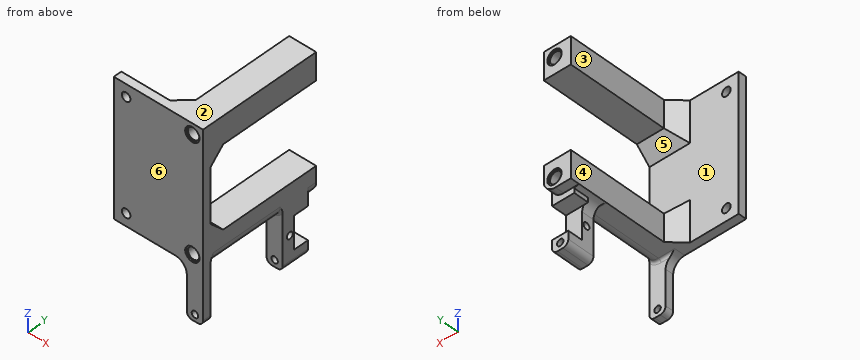
```python
from build123d import *

# Parameters (mm, degrees)
SKETCH1_R           = 1.5999999999999974
SKETCH1_R_2         = 1.6
BOSS_EXTRUDE1_DEPTH = 3
SKETCH2_W           = 10.000000000000004
SKETCH2_H           = 10.000000000000004
BOSS_EXTRUDE2_DEPTH = 42
CHAMFER1_SIZE       = 5
SKETCH3_R           = 2.1
SKETCH3_R_2         = 2.1000000000000005
CUT_EXTRUDE1_DEPTH  = 52.00000000000001
SKETCH4_R           = 2.65
SKETCH4_R_2         = 2.6500000000000004
CUT_EXTRUDE2_DEPTH  = 0.5
BOSS_EXTRUDE3_DEPTH = 14.15
SKETCH6_R           = 1.2000000000000004
CUT_EXTRUDE3_DEPTH  = 6
SKETCH7_W           = 6
SKETCH7_H           = 10.018921584932333
BOSS_EXTRUDE4_DEPTH = 5
BOSS_EXTRUDE5_DEPTH = 2.15
SKETCH9_W           = 6
SKETCH9_H           = 3
BOSS_EXTRUDE6_DEPTH = 19.15
SKETCH10_R          = 1.2000000000000004
CUT_EXTRUDE4_DEPTH  = 64.7666045986287
FILLET3_R           = 2
FILLET4_R           = 4.25
FILLET5_R           = 4.25
FILLET6_R           = 4.25
FILLET7_R           = 4.25
FILLET8_R           = 1
FILLET9_R           = 1


with BuildPart() as part:
    # Sketch1 → Boss-Extrude1 (new body)
    with BuildSketch(Plane(origin=(0, 0, 0), x_dir=(1, 0, 0), z_dir=(0, 1, 0))):
        Polygon((-6.5123966942148765, 9.68595041322314), (1.487603305785124, 9.68595041322314), (26.48760330578513, 9.68595041322314), (26.487603305785132, -40.31404958677687), (1.4876033057851312, -40.31404958677687), (-6.512396694214871, -40.31404958677687), align=None)
        with Locations(Location((-1.962396694214872, -35.76404958677687, 0), (0, 0, 270))):
            Circle(SKETCH1_R, mode=Mode.SUBTRACT)
        with Locations(Location((-1.9623966942148756, 5.135950413223139, 0), (0, 0, 270))):
            Circle(SKETCH1_R_2, mode=Mode.SUBTRACT)
    extrude(amount=BOSS_EXTRUDE1_DEPTH)

    # Sketch2 → Boss-Extrude2 (add)
    with BuildSketch(Plane(origin=(0, 3, 0), x_dir=(1, 0, 0), z_dir=(0, 1, 0))):
        with Locations((21.48760330578513, -35.31404958677687)):
            Rectangle(SKETCH2_W, SKETCH2_H)
        Polygon((26.48760330578513, 9.68595041322314), (16.48760330578513, 9.685950413223138), (16.487603305785125, -0.314049586776863), (26.48760330578513, -0.31404958677686173), align=None)
    extrude(amount=BOSS_EXTRUDE2_DEPTH)

    # Chamfer1
    chamfer1_edges = [part.edges().sort_by_distance(p)[0] for p in [
        (21.48760330578513, 3, 30.314049586776864),
        (16.48760330578513, 3, 35.31404958677687),
        (16.48760330578513, 3, -4.6859504132231375),
        (21.48760330578513, 3, 0.31404958677686234),
    ]]
    chamfer(chamfer1_edges, length=CHAMFER1_SIZE)

    # Sketch3 → Cut-Extrude1 (cut)
    with BuildSketch(Plane(origin=(0, 45.00000000000001, 0), x_dir=(1, 0, 0), z_dir=(0, 1, 0))):
        with Locations(Location((22.53760330578513, -36.364049586776865, 0), (0, 0, 270))):
            Circle(SKETCH3_R)
        with Locations(Location((22.53760330578513, 5.735950413223138, 0), (0, 0, 270))):
            Circle(SKETCH3_R_2)
    extrude(amount=-CUT_EXTRUDE1_DEPTH, mode=Mode.SUBTRACT)

    # Sketch4 → Cut-Extrude2 (cut)
    with BuildSketch(Plane(origin=(0, 45.00000000000001, 0), x_dir=(1, 0, 0), z_dir=(0, 1, 0))):
        with Locations(Location((22.53760330578513, -36.364049586776865, 0), (0, 0, 270))):
            Circle(SKETCH4_R)
        with Locations(Location((22.53760330578513, 5.735950413223138, 0), (0, 0, 270))):
            Circle(SKETCH4_R_2)
    cut_extrude2 = extrude(amount=-CUT_EXTRUDE2_DEPTH, mode=Mode.SUBTRACT)

    # Mirror1: Cut-Extrude2 across plane
    add(cut_extrude2.mirror(Plane(origin=(0, 22.500000000000004, 0), x_dir=(0, 0, 1), z_dir=(0, -1, 0))), mode=Mode.SUBTRACT)

    # Sketch5 → Boss-Extrude3 (add)
    with BuildSketch(Plane(origin=(0, 0, -9.68595041322314), x_dir=(-1, 0, 0), z_dir=(0, 0, -1))):
        Polygon((-20.487603305785136, 36.20000000000077), (-26.487603305785136, 36.20000000000077), (-26.487603305785132, 31.68676314830412), (-20.487603305785132, 31.68676314830412), align=None)
    extrude(amount=BOSS_EXTRUDE3_DEPTH)

    # Sketch6 → Cut-Extrude3 (cut)
    with BuildSketch(Plane(origin=(26.48760330578513, 0, -1.84e-15), x_dir=(0, 0, -1), z_dir=(1, -7.7e-16, 0))):
        with Locations(Location((17.835950413222832, 34.50000000000082, 0), (0, 0, 90))):
            Circle(SKETCH6_R)
    extrude(amount=-CUT_EXTRUDE3_DEPTH, mode=Mode.SUBTRACT)

    # Sketch7 → Boss-Extrude4 (add)
    with BuildSketch(Plane(origin=(1.35e-15, 1.098e-14, -23.835950413222633), x_dir=(-1, 0, -6e-17), z_dir=(6e-17, 4.6e-16, -1))):
        with Locations((-23.487603305785132, 36.696223940770274)):
            Rectangle(SKETCH7_W, SKETCH7_H)
    extrude(amount=BOSS_EXTRUDE4_DEPTH)

    # Sketch8 → Boss-Extrude5 (add)
    with BuildSketch(Plane(origin=(0, 0, -9.68595041322314), x_dir=(-1, 0, 0), z_dir=(0, 0, -1))):
        Polygon((-26.487603305785136, 36.20000000000077), (-18.268679093182527, 36.2000000000008), (-18.268679093182527, 41.70568473323645), (-26.487603305785136, 41.70568473323645), align=None)
    extrude(amount=BOSS_EXTRUDE5_DEPTH)

    # Sketch9 → Boss-Extrude6 (add)
    with BuildSketch(Plane(origin=(0, 0, -9.68595041322314), x_dir=(-1, 0, 0), z_dir=(0, 0, -1))):
        with Locations((-23.487603305785132, 1.5)):
            Rectangle(SKETCH9_W, SKETCH9_H)
    extrude(amount=BOSS_EXTRUDE6_DEPTH)

    # Sketch10 → Cut-Extrude4 (cut, through all)
    with BuildSketch(Plane(origin=(0, 41.70568473323644, 1.921e-14), x_dir=(1, 0, 0), z_dir=(0, 1, 4.6e-16))):
        with Locations(Location((23.487603305785132, 26.335950413222633, 0), (0, 0, 270))):
            Circle(SKETCH10_R)
    extrude(amount=-CUT_EXTRUDE4_DEPTH, mode=Mode.SUBTRACT)

    # Fillet3
    fillet3_edges = [part.edges().sort_by_distance(p)[0] for p in [
        (26.487603305785132, 36.69622394077029, -28.835950413222616),
        (20.487603305785132, 36.69622394077029, -28.835950413222616),
        (20.487603305785132, 1.5, -28.835950413223138),
        (26.487603305785132, 1.5, -28.835950413223138),
    ]]
    fillet(fillet3_edges, radius=FILLET3_R)

    # Fillet4
    fillet4_edges = [part.edges().sort_by_distance(p)[0] for p in [
        (26.48760330578513, 17.343381574152062, -9.68595041322314),
    ]]
    fillet(fillet4_edges, radius=FILLET4_R)

    # Fillet5
    fillet5_edges = [part.edges().sort_by_distance(p)[0] for p in [
        (20.487603305785132, 1.5, -9.68595041322314),
    ]]
    fillet(fillet5_edges, radius=FILLET5_R)

    # Fillet6
    fillet6_edges = [part.edges().sort_by_distance(p)[0] for p in [
        (26.48760330578513, 43.352842366618226, -9.68595041322314),
    ]]
    fillet(fillet6_edges, radius=FILLET6_R)

    # Fillet7
    # the kernel refuses this fillet: 4.25 mm, written as the material it adds along each edge
    with BuildSketch(Plane(origin=(20.487603305785132, 31.68676314830412, -9.68595041322314), x_dir=(-1, 7.9e-16, 8.9e-16), z_dir=(7.9e-16, 1, 0))) as fillet7_piece_1:
        with BuildLine():
            CenterArc((4.2499999999999964, -4.242640687119286), FILLET7_R, 93.37228668343381, 86.62771331656613)
            Line((-3.77e-15, -4.242640687119282), (0, 0))
            Line((0, 0), (4.0000000000000036, 0))
        make_face()
    extrude(amount=4.51323685169665)
    with BuildSketch(Plane(origin=(20.48760330578512, 21.08016143050591, -9.68595041322314), x_dir=(-1, 7.9e-16, 0), z_dir=(7.9e-16, 1, 0))) as fillet7_piece_2_section:
        with BuildLine():
            CenterArc((4.2499999999999964, -4.242640687119284), FILLET7_R, 93.37228668343396, 86.62771331656604)
            Line((-3.55e-15, -4.242640687119284), (0, 0))
            Line((0, 0), (3.999999999999993, 0))
        make_face()
    fillet7_piece_2 = extrude(amount=25.726440287293073, mode=Mode.PRIVATE)
    fillet7_piece_2 = split(fillet7_piece_2, bisect_by=Plane(origin=(17.40856960112635, 36.2000000000008, -9.834246197287131), z_dir=(3.46e-15, 1, 0)), keep=Keep.TOP, mode=Mode.PRIVATE)
    fillet7_piece_2 = split(fillet7_piece_2, bisect_by=Plane(origin=(18.268679093182527, 38.95284236661862, -9.834246197287131), z_dir=(-1, 0, 0)), keep=Keep.TOP, mode=Mode.PRIVATE)
    fillet7_piece_2 = split(fillet7_piece_2, bisect_by=Plane(origin=(17.40856960112636, 41.70568473323645, -9.834246197287131), z_dir=(0, -1, 0)), keep=Keep.TOP, mode=Mode.PRIVATE)
    add(fillet7_piece_2)

    # Fillet8
    fillet8_edges = [part.edges().sort_by_distance(p)[0] for p in [
        (19.23760330578513, 3, -9.68595041322314),
        (25.242807125827955, 3, -8.441154233265967),
    ]]
    fillet(fillet8_edges, radius=FILLET8_R)

    # Fillet9
    # the kernel refuses this fillet: 1 mm, written as the material it adds along each edge
    with BuildSketch(Plane(origin=(22.23760330578513, 31.68676314830412, -9.68595041322314), x_dir=(2.101e-14, -1, 0), z_dir=(-1, -2.101e-14, 4.881e-14))) as fillet9_piece_1_section:
        with BuildLine():
            CenterArc((FILLET9_R, -FILLET9_R), FILLET9_R, 90, 90)
            Line((0, -FILLET9_R), (0, 0))
            Line((0, 0), (FILLET9_R, 0))
        make_face()
    fillet9_piece_1 = extrude(amount=5.750000000000124, mode=Mode.PRIVATE)
    fillet9_piece_1 = fillet9_piece_1 - Plane(origin=(16.237603305785, 31.449849305224696, -13.928591100342), x_dir=(-1, 0, 0), z_dir=(0, -1, 0)) * Cylinder(4.25, 16, mode=Mode.PRIVATE)
    add(fillet9_piece_1)
    with BuildSketch(Plane(origin=(22.23760330578513, 31.68676314830412, -5.43595041322314), x_dir=(0, 0, -1), z_dir=(-1, 0, 0))) as fillet9_piece_2_section:
        with BuildLine():
            CenterArc((4.249999999999999 + FILLET9_R, FILLET9_R), FILLET9_R, 180.00000000000693, 89.99999999999307)
            Line((4.249999999999999, FILLET9_R), (4.249999999999999, 0))
            Line((4.249999999999999, 0), (4.249999999999999 + FILLET9_R, 1.2079e-13))
        make_face()
    fillet9_piece_2 = revolve(axis=Axis((22.23760330578513, 31.68676314830412, -5.43595041322314), (0, -1, 0)), revolution_arc=123.71693864409282, mode=Mode.PRIVATE)
    fillet9_piece_2 = split(fillet9_piece_2, bisect_by=Plane(origin=(26.48760330578513, 31.521836885030236, -9.895455596994594), z_dir=(-1, 0, 7e-17)), keep=Keep.TOP, mode=Mode.PRIVATE)
    add(fillet9_piece_2)


solid = part.part
```
Design review of the part built by this model. Coordinates are the model's own, in mm. Face numbers are marked on the shaded views. A direction names the side the tool comes from. Coordinates: 2 decimals unless noted, no trailing zeros. Order: outer loops, then holes, each group sorted by start corner. A loop starts at its lowest first (then second) coordinate and runs counter-clockwise, first axis right, second up.
1) Clearance check with flat-ended pins moving along their axes: pin 1 (6.5 mm diameter, centred on x = 22.54, z = 36.36, fed in from +Y); pin 2 (4 mm diameter, centred on x = -2, z = 10, fed in from +Y); pin 3 (1.6 mm diameter, centred on x = 18.5, y = 43, fed in from -Z); pin 4 (4 mm diameter, centred on x = 23, z = 36.5, fed in from -Y). State where each tip first meets the part, or that it passes through.
2) For the marked faces 4, 5 and 6, list the 3-axis set-ups (+Z, -Z, +X, -X, +Y, -Y) from which the entire face can be reached by the end or side of a thin tool; tool diameter is ignored.
3) Wall thickness on line 1 along Z through (x, y) = (21, 9); line 2 along Y through (x, z) = (11, 26.5); line 3 along Y through (x, z) = (24, -20): over which ranges is each line inside the solid? List them lowest first.
4) Take a section at D-D, the plane x = 4. Give the boundary of the cut face in (y, z), and give its area (3 significant figures).
5) Mouldability with a two-part tool opening along Z and no side actions: class the marked faces 1, 2 and 3 as +Z half, -Z half, draft (parallel to the pull), parting line (faces both ways), or undercut.
6) Take a section at B-B, the plane y = 34.5. Give the boundary of the cut face in (x, z).
7) Take a section at C-C, the plane x = 12.5. Give the boundary of the cut face in (y, z), and give its area (3 significant figures).
8) Take a section at A-A, the plane y = 14. Give the boundary of the cut face in (x, z), and give its area (3 significant figures).
Returned:
1. pin 1: stops at y = 45
1. pin 2: stops at y = 3
1. pin 3: stops at z = -9.69
1. pin 4: stops at y = 0.5
2. face 4: +Z, -Z, -X, +Y
2. face 5: +X, -X, +Y
2. face 6: +Z, -Z, +X, -X, -Y
3. line 1: z = -9.69 to -7.17, -4.31 to 0.31, 30.31 to 34.93, 37.79 to 40.31
3. line 2: y = 0 to 3
3. line 3: y = 0 to 3, 31.69 to 36.2
4. outline: (0, -9.69) - (3, -9.69) - (3, 40.31) - (0, 40.31) - close
4. area: 150 mm2
5. face 1: undercut
5. face 2: +Z half
5. face 3: draft
6. outline: (16.49, -9.69) arc R4.25 cw to (20.49, -13.93) - (20.49, -16.64) - (26.49, -16.64) - (26.49, 0.31) - (16.49, 0.31) - close; (16.49, 30.31) - (26.49, 30.31) - (26.49, 40.31) - (16.49, 40.31) - close; (20.49, -26.84) arc R2 ccw to (22.49, -28.84) - (24.49, -28.84) arc R2 ccw to (26.49, -26.84) - (26.49, -19.04) - (20.49, -19.04) - close; hole circle Ø4.2 at (22.54, -5.74); hole circle Ø4.2 at (22.54, 36.36); hole circle Ø2.4 at (23.49, -26.34)
7. outline: (0, -9.69) - (4.01, -9.69) - (4.01, 4.3) - (3, 5.31) - (3, 25.31) - (4.01, 26.33) - (4.01, 40.31) - (0, 40.31) - close
7. area: 179 mm2
8. outline: (16.49, -9.69) - (22.24, -9.69) arc R4.25 ccw to (26.49, -5.44) - (26.49, 0.31) - (16.49, 0.31) - close; (16.49, 30.31) - (26.49, 30.31) - (26.49, 40.31) - (16.49, 40.31) - close; hole circle Ø4.2 at (22.54, -5.74); hole circle Ø4.2 at (22.54, 36.36)
8. area: 168 mm2
